Part model, mm, in its own coordinate system. Face numbers are marked on the shaded views. A direction names the side the tool comes from. Give positions to 0.01 mm unless a question says otherwise; leave off trailing zeros. Write each loop counter-clockwise with the first axis right and the second up, starting at its lowest first coordinate (ties: lowest second). Pieces come first, ordered by that corner, then holes.
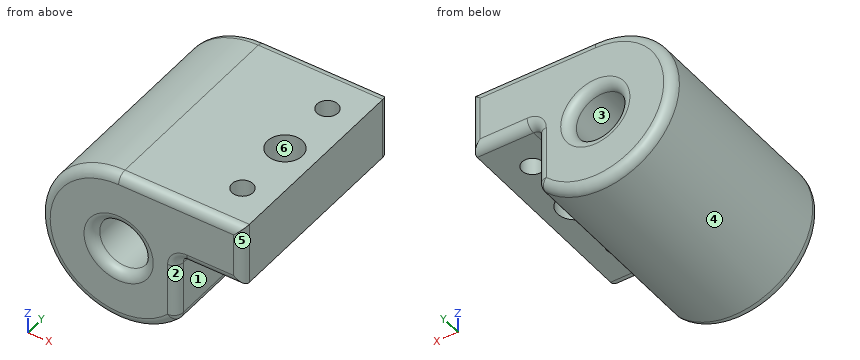
from build123d import *

# Parameters (mm, degrees)
F0_R     = 4.1275
F1_DEPTH = 34.925
F2_R     = 2.8575
F2_R_2   = 1.7145
F3_DEPTH = 25.4
F4_R     = 1.6002
F5_R     = 1.524
F6_R     = 1.524
F7_R     = 1.524


with BuildPart() as f1:
    # F0 (on Front) → F1 (new body)
    with BuildSketch(Plane.XZ):
        with BuildLine():
            Line((20.32, 12.7), (0, 12.7))
            ThreePointArc((0, 12.7), (-11.57526, -5.22526), (9.525, -8.40026))
            Line((9.525, -8.40026), (9.525, 2.54))
            Line((9.525, 2.54), (12.443408, 2.54))
            Line((12.443408, 2.54), (20.32, 2.54))
            Line((20.32, 2.54), (20.32, 12.7))
        make_face()
        Circle(F0_R, mode=Mode.SUBTRACT)
    extrude(amount=F1_DEPTH)

    # F2 (on face) → F3 (cut)
    with BuildSketch(Plane.XY.offset(12.7)):
        with Locations((15.24, -17.4625)):
            Circle(F2_R)
        with Locations((15.24, -27.6225)):
            Circle(F2_R_2)
        with Locations((15.24, -7.3025)):
            Circle(F2_R_2)
    extrude(amount=-F3_DEPTH, mode=Mode.SUBTRACT)

    # F4
    f4_edges = [f1.edges().sort_by_distance(p)[0] for p in [
        (9.525, -17.4625, 2.54),
    ]]
    fillet(f4_edges, radius=F4_R)

    # F5
    f5_edges = [f1.edges().sort_by_distance(p)[0] for p in [
        (9.525, -34.925, -3.73023),
        (9.993688, -34.925, 2.071312),
        (-11.57526, -34.925, -5.22526),
        (15.7226, -34.925, 2.54),
        (10.16, -34.925, 12.7),
        (20.32, -34.925, 7.62),
        (-4.1275, -34.925, 0),
    ]]
    fillet(f5_edges, radius=F5_R)

    # F6
    f6_edges = [f1.edges().sort_by_distance(p)[0] for p in [
        (9.525, 0, -3.73023),
        (9.993688, 0, 2.071312),
        (-11.57526, 0, -5.22526),
        (15.7226, 0, 2.54),
        (10.16, 0, 12.7),
        (20.32, 0, 7.62),
        (-4.1275, 0, 0),
    ]]
    fillet(f6_edges, radius=F6_R)

    # F7
    f7_edges = [f1.edges().sort_by_distance(p)[0] for p in [
        (9.525, -17.4625, -8.40026),
    ]]
    fillet(f7_edges, radius=F7_R)


solid = f1.part
1) Flat gauge pins, fed straight in: P1, Ø3, axis at x = 17.5, y = -14.5, coming from the -Z side; P2, Ø6, axis at y = -14.5, z = 7, coming from the -X side; P3, Ø1, axis at y = -24.5, z = -5.5, coming from the -X side. Where does each tip first touch, or does it go through?
Check result:
P1: stops at z = 2.54
P2: stops at x = -12.05
P3: stops at x = -11.67
2) Saw through at A-A (y = -4). Write the cut outline in (x, z) (1 decimal).
Check result:
outline: (0, 12.7) arc R12.7 ccw (long way) to (9.1, -8.9) arc R1.5 ccw to (9.5, -7.8) - (9.5, 0.9) arc R1.6 cw to (11.1, 2.5) - (20.3, 2.5) - (20.3, 12.7) - close; hole circle Ø8.3 at (0, 0)
3) Saw through at B-B (x = 15.24). Write the cut outline in (y, z) (3 decimals).
Check result:
outline: (-34.925, 4.064) arc R1.524 ccw to (-33.401, 2.54) - (-29.337, 2.54) - (-29.337, 12.7) - (-33.401, 12.7) arc R1.524 ccw to (-34.925, 11.176) - close; (-25.908, 2.54) - (-20.32, 2.54) - (-20.32, 12.7) - (-25.908, 12.7) - close; (-14.605, 2.54) - (-9.017, 2.54) - (-9.017, 12.7) - (-14.605, 12.7) - close; (-5.588, 2.54) - (-1.524, 2.54) arc R1.524 ccw to (0, 4.064) - (0, 11.176) arc R1.524 ccw to (-1.524, 12.7) - (-5.588, 12.7) - close
4) Drill centre lines: L1, parallel to Y at x = 15.24, z = 9 (3 decimals); L2, parallel to Z at x = 0, y = -25.5; L3, parallel to Z at x = 1.5, y = -20. Where is each one in solid material? Low to high.
Check result:
L1: y = -34.925 to -29.337, -25.908 to -20.32, -14.605 to -9.017, -5.588 to 0
L2: z = -12.7 to -4.13, 4.13 to 12.7
L3: z = -12.61 to -3.85, 3.85 to 12.7
5) 3-axis set-ups, long thin cutter, end or side, ignore diameter. For the marked faces 1, 2 and 3: which of +Z, -Z, +X, -X, +Y, -Y reach the whole face in a straight line?
Check result:
face 1: -Z, +X, +Y, -Y
face 2: -Z, +X, -Y
face 3: +Y, -Y
6) Saw through at C-C (z = 3.5). State how many separate pieces and enclosed holes the cut face has, and give its area (3 significant figures).
Check result:
separate pieces: 2
enclosed holes: 3
area: 932 mm2
7) Mould opens along Y. For the marked faces 4, 5 and 6 say: +Y half, -Y half, draft (parallel to the pull), parting line (faces both ways), or undercut.
Check result:
face 4: draft
face 5: -Y half
face 6: undercut
